Input: part model. Units: mm. Frame: model coordinates. Face numbers are marked on the shaded views. A direction names the side the tool comes from. Give positions to 0.01 mm unless a question says otherwise; leave off trailing zeros. Loops run counter-clockwise (first coordinate to the right, second up) from the corner with the lowest first, then second, coordinate; pieces in that order, holes last. Notation, with made-up numbers: M -38,-6.75 L 21,-6.75 A9 ccw 21,7.25 Z; hole C 19,36 d7. An arc over 180 degrees is marked long. Answer as a JSON object with one key per item and string values. Group by question number.
1) Section query B-B on x = 1.75. Return loops of the section in (y, z).
2) Access query for the marked faces 4 and 5. Directions: +Z, -Z, +X, -X, +Y, -Y. A direction counts if a zero-diameter tool reaches every point of the face in a straight line with its end or side. Return the directions, or none.
3) Ray query, L1, parallel to X at y = 15, z = 6.25; L2, parallel to X at y = -2.5, z = 0; L3, parallel to Y at x = 0, z = 5.65. Return the intervals inside material, ascending.
4) First-contact query: P1, Ø8, axis at x = 3, y = -12, coming from the +Z side; P2, Ø8, axis at y = -13, z = -1, coming from the -X side; P3, Ø3, axis at y = 15.5, z = 3, coming from the -X side; P4, Ø3, axis at y = 14, z = 9, coming from the +X side. Flat tips, straight axial feed; report the tip coordinate or a pass-through.
5) Draft query along X for the marked faces 1, 2 and 3. Return one class per face: +X half, -X half, draft (parallel to the pull), parting line (faces both ways), or undercut.
6) Section query D-D on z = 4.5. Return loops of the section in (x, y).
7) Section query A-A on z = 0. Return loops of the section in (x, y), plus the area to 3 significant figures.
8) Section query C-C on y = 15. Return loops of the section in (x, z), plus the area to 3 significant figures.
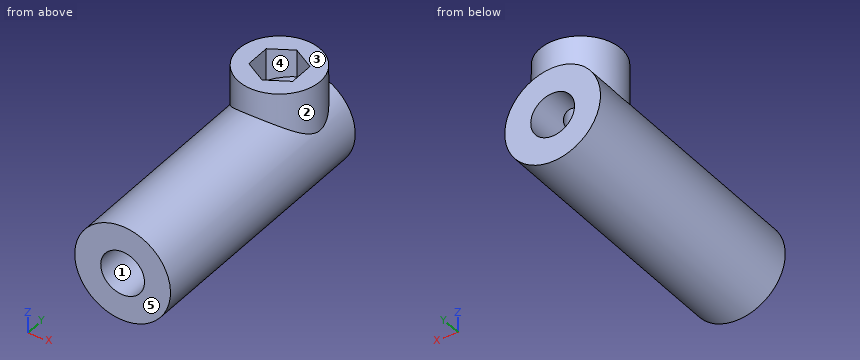
from build123d import *

# Parameters (mm, degrees)
CROQUIS1_R                   = 7.65
SALIENTE_EXTRUIR1_DEPTH      = 8.5
CROQUIS2_R                   = 7.65
CROQUIS2_R_2                 = 3.5
SALIENTE_EXTRUIR2_DEPTH      = 21.5
SALIENTE_EXTRUIR3_REACH      = 132.896
SALIENTE_EXTRUIR3_END_RADIUS = 7.65
SALIENTE_EXTRUIR3_START      = 12
CROQUIS3_R                   = 6.5
CORTAR_EXTRUIR1_REACH        = 129.309
CORTAR_EXTRUIR1_END_RADIUS   = 3.5
CROQUIS4_R                   = 2.25


with BuildPart() as part:
    # Croquis1 → Saliente-Extruir1 (new, symmetric)
    with BuildSketch(Plane(origin=(0, 0, 0), x_dir=(1, 0, 0), z_dir=(0, 1, 0))):
        with BuildLine():
            ThreePointArc((-18.62950636, 70.733830846), (-21.266037972, 78.379045573), (-29.224003483, 79.818278736))
            ThreePointArc((-29.224003483, 79.818278736), (-42.5, 73.612159322), (-54.51265533, 65.217868785))
            ThreePointArc((-54.51265533, 65.217868785), (-57.245225604, 57.606451909), (-51.942541239, 51.500541191))
            ThreePointArc((-51.942541239, 51.500541191), (-41.569219382, 24), (-70.572047599, 19.233289655))
            ThreePointArc((-70.572047599, 19.233289655), (-78.511263577, 20.772593665), (-83.736658814, 14.600409951))
            ThreePointArc((-83.736658814, 14.600409951), (-85, 0), (-83.736658814, -14.600409951))
            ThreePointArc((-83.736658814, -14.600409951), (-78.511263577, -20.772593665), (-70.572047599, -19.233289655))
            ThreePointArc((-70.572047599, -19.233289655), (-41.569219382, -24), (-51.942541239, -51.500541191))
            ThreePointArc((-51.942541239, -51.500541191), (-57.245225604, -57.606451909), (-54.51265533, -65.217868785))
            ThreePointArc((-54.51265533, -65.217868785), (-42.5, -73.612159322), (-29.224003483, -79.818278736))
            ThreePointArc((-29.224003483, -79.818278736), (-21.266037972, -78.379045573), (-18.62950636, -70.733830846))
            ThreePointArc((-18.62950636, -70.733830846), (0, -48), (18.62950636, -70.733830846))
            ThreePointArc((18.62950636, -70.733830846), (21.266037972, -78.379045573), (29.224003483, -79.818278736))
            ThreePointArc((29.224003483, -79.818278736), (42.5, -73.612159322), (54.51265533, -65.217868785))
            ThreePointArc((54.51265533, -65.217868785), (57.245225604, -57.606451909), (51.942541239, -51.500541191))
            ThreePointArc((51.942541239, -51.500541191), (41.569219382, -24), (70.572047599, -19.233289655))
            ThreePointArc((70.572047599, -19.233289655), (78.511263577, -20.772593665), (83.736658814, -14.600409951))
            ThreePointArc((83.736658814, -14.600409951), (85, 0), (83.736658814, 14.600409951))
            ThreePointArc((83.736658814, 14.600409951), (78.511263577, 20.772593665), (70.572047599, 19.233289655))
            ThreePointArc((70.572047599, 19.233289655), (41.569219382, 24), (51.942541239, 51.500541191))
            ThreePointArc((51.942541239, 51.500541191), (57.245225604, 57.606451909), (54.51265533, 65.217868785))
            ThreePointArc((54.51265533, 65.217868785), (42.5, 73.612159322), (29.224003483, 79.818278736))
            ThreePointArc((29.224003483, 79.818278736), (21.266037972, 78.379045573), (18.62950636, 70.733830846))
            ThreePointArc((18.62950636, 70.733830846), (0, 48), (-18.62950636, 70.733830846))
        make_face()
        with Locations(Location((0, 0, 0), (0, 0, 270))):
            Circle(CROQUIS1_R, mode=Mode.SUBTRACT)
    extrude(amount=SALIENTE_EXTRUIR1_DEPTH, both=True)


with BuildPart() as body_2:
    # Croquis2 → Saliente-Extruir2 (new body)
    with BuildSketch(Plane(origin=(0, 0, 0), x_dir=(1, 0, 0), z_dir=(0, 1, 0))):
        with Locations(Location((0, 0, 0), (0, 0, 270))):
            Circle(CROQUIS2_R)
        with Locations(Location((0, 0, 0), (0, 0, 270))):
            Circle(CROQUIS2_R_2, mode=Mode.SUBTRACT)
    extrude(amount=SALIENTE_EXTRUIR2_DEPTH)

    # Simetría3: body 2 across plane


with BuildPart() as body_2_1:
    add(body_2.part)
    add(body_2.part.mirror(Plane.ZX))

    # Saliente-Extruir3: up to this cylinder (the profile starts outside it)
    saliente_extruir3_end = Plane(origin=(0, 15, 0), z_dir=(0, -1, 0)) * Cylinder(SALIENTE_EXTRUIR3_END_RADIUS, 282.092, mode=Mode.PRIVATE)
    # Croquis3 → Saliente-Extruir3 (add, up to the surface)
    with BuildSketch(Plane.XY.offset(SALIENTE_EXTRUIR3_START), mode=Mode.PRIVATE) as saliente_extruir3_sk1:
        with Locations((0, 15)):
            Circle(CROQUIS3_R)
        Polygon((0, 10.958548116), (3.5, 12.979274058), (3.5, 17.020725942), (0, 19.041451884), (-3.5, 17.020725942), (-3.5, 12.979274058), align=None, mode=Mode.SUBTRACT)
    saliente_extruir3_tool1 = extrude(saliente_extruir3_sk1.sketch, amount=-SALIENTE_EXTRUIR3_REACH, mode=Mode.PRIVATE) - saliente_extruir3_end
    add(saliente_extruir3_tool1.solids().sort_by_distance((-6.316152, 15, 12))[0])

    # Cortar-Extruir1: up to this cylinder (the profile starts outside it)
    cortar_extruir1_end = Plane(origin=(0, 15, 0), z_dir=(0, -1, 0)) * Cylinder(CORTAR_EXTRUIR1_END_RADIUS, 266.618, mode=Mode.PRIVATE)
    # Croquis4 → Cortar-Extruir1 (cut, up to the surface)
    with BuildSketch(Plane.XY.offset(12), mode=Mode.PRIVATE) as cortar_extruir1_sk1:
        with Locations((0, 15)):
            Circle(CROQUIS4_R)
    cortar_extruir1_tool1 = extrude(cortar_extruir1_sk1.sketch, amount=-CORTAR_EXTRUIR1_REACH, mode=Mode.PRIVATE) - cortar_extruir1_end
    add(cortar_extruir1_tool1.solids().sort_by_distance((0, 15, 12))[0], mode=Mode.SUBTRACT)


solid = body_2_1.part
Output:
{
 "1": {"outline": "M -21.5,-7.45 L 21.5,-7.45 L 21.5,-3.03 L -21.5,-3.03 Z; M -21.5,3.03 L 13.59,3.03 L 13.59,7.45 L 11.97,7.45 L 11.97,12 L 8.74,12 L 8.74,7.45 L -21.5,7.45 Z; M 16.41,3.03 L 21.5,3.03 L 21.5,7.45 L 21.26,7.45 L 21.26,12 L 18.03,12 L 18.03,7.45 L 16.41,7.45 Z"},
 "2": {"face 4": "+Z", "face 5": "+Z, -Z, +X, -X, -Y"},
 "3": {"L1": "x = -6.5 to -2.25, 2.25 to 6.5", "L2": "x = -7.65 to -3.5, 3.5 to 7.65", "L3": "y = -21.5 to 12.75, 17.25 to 21.5"},
 "4": {"P1": "stops at z = 7.65", "P2": "stops at x = -7.65", "P3": "stops at x = -7.5", "P4": "stops at x = 6.5"},
 "5": {"face 1": "undercut", "face 2": "parting line", "face 3": "draft"},
 "6": {"outline": "M -6.19,-21.5 L 6.19,-21.5 L 6.19,13.01 A6.5 ccw 6.19,16.99 L 6.19,21.5 L -6.19,21.5 L -6.19,16.99 A6.5 ccw -6.19,13.01 Z; hole C 0,15 d4.5"},
 "7": {"outline": "M -7.65,-21.5 L -3.5,-21.5 L -3.5,21.5 L -7.65,21.5 Z; M 3.5,-21.5 L 7.65,-21.5 L 7.65,21.5 L 3.5,21.5 Z", "area": "357 mm^2"},
 "8": {"outline": "M -6.5,4.03 A7.65 ccw long 6.5,4.03 L 6.5,12 L 3.5,12 L 3.5,6.8 A7.65 ccw 2.25,7.31 L 2.25,2.68 A3.5 cw long -2.25,2.68 L -2.25,7.31 A7.65 ccw -3.5,6.8 L -3.5,12 L -6.5,12 Z", "area": "164 mm^2"}
}
